Build history of the part. All positions in model axes, mm. A direction names the side the tool comes from. Give positions to 0.01 mm unless a question says otherwise; leave off trailing zeros. Order: outer loops, then holes, each group sorted by start corner. A loop starts at its lowest first (then second) coordinate and runs counter-clockwise, first axis right, second up. Notation, with made-up numbers: (20, 66) - (66, 66) arc R31 ccw to (66, 105) - close; hole circle Ø6 at (76.5, 54.25). An arc over 180 degrees is marked (long way). Use a Markdown table: item, result.
Autodesk Inventor part; units mm, degrees
ref_plane "Work Plane1" through (-19.467767, 1.0375, -4.375) normal (0, 0, -1) x (0, 1, 0)
ref_plane "YZ Plane" through (0, 0, 0) normal (1, 0, 0) x (0, 1, 0)
ref_plane "XZ Plane" through (0, 0, 0) normal (0, 1, 0) x (-1, 0, 0)
sketch "Sketch1" plane through (0, 0, 0) normal (0, 0, 1) x (1, 0, 0)
  circle A0 centre (1.767767, 26.667767) radius 7
  circle A1 centre (1.767767, 26.667767) radius 6.965
  circle A2 centre (1.767767, 26.667767) radius 6.09
  point P0 (0, 0)
  dimension "d0" = 0.035
  dimension "d2" = 0.875
ref_plane "Work Plane1" through (-19.467767, 1.0375, -4.375) normal (0, 0, -1) x (0, 1, 0)
sketch "Sketch1 outline for Extrusion1" plane through (0, 0, 0) normal (0, 0, 1) x (1, 0, 0)
  circle A0 centre (1.767767, 26.667767) radius 6.965
  circle A1 centre (1.767767, 26.667767) radius 6.09
extrude "Extrusion1" add sketch "Sketch1 outline for Extrusion1" along normal blind 1.25 from surface at -4.375
sketch "Sketch2" plane through (1.767767, 26.667767, -4.375) normal (0, 0, -1) x (-1, 0, 0)
  circle A0 centre (0, 0) radius 6.965
  circle A1 centre (0, 0) radius 6.09
  circle A2 centre (0, 0) radius 7.09
  circle A3 centre (0, 0) radius 9.09
  point P0 (1.767767, -26.667767)
  dimension "d5" = 0.125
  dimension "d6" = 2
extrude "Extrusion2" add sketch "Sketch2" along normal blind 1.25 contours A0 | A2 | A3
properties part number "Half Inch Lense Holder Cover (V5)"
1) Slice it at B-B (x = -2.5). Write the cut outline in (y, z) (3 decimals).
Computed:
| item | result |
|---|---|
| outline | (18.642, -5.625) - (22.323, -5.625) - (22.323, -3.125) - (21.163, -3.125) - (21.163, -4.375) - (18.642, -4.375) - close; (31.012, -5.625) - (34.694, -5.625) - (34.694, -4.375) - (32.172, -4.375) - (32.172, -3.125) - (31.012, -3.125) - close |
2) Tool access for faces 1 (the flat face through (6, 22, -3.125)), 2 (the flat face through (-3, 21, -4.375)): list every direction of +Z, -Z, +X, -X, +Y, -Y with a clear straight run to the whole face (end or side of a thin tool).
Computed:
| item | result |
|---|---|
| face 1 | +Z, +X, -X, +Y, -Y |
| face 2 | +Z |
3) Slice it at C-C (x = 8.25). Write the cut outline in (y, z) (3 decimals).
Computed:
| item | result |
|---|---|
| outline | (20.295, -5.625) - (33.04, -5.625) - (33.04, -4.375) - (29.216, -4.375) - (29.216, -3.125) - (24.12, -3.125) - (24.12, -4.375) - (20.295, -4.375) - close |
4) Wall check: line 1 (X direction, y = 26.5, z = -3.75); line 2 (Z direction, x = 8, y = 32) (3 decimals); line 3 (Y direction, x = 5.5, z = -5.15). Give the ranges that are in metal, low to high. Write a range as from..to.
Computed:
| item | result |
|---|---|
| line 1 | x = -5.2..-4.32, 7.86..8.73 |
| line 2 | z = -5.625..-4.375 |
| line 3 | y = 18.38..21.86, 31.48..34.96 |
5) Pin check, flat tips, straight feed: P1, Ø1, axis at x = 9, z = -5, coming from the +Y side; P2, Ø9.5, axis at x = 1.77, y = 26.67, coming from the +Z side; P3, Ø10, axis at x = 7, y = 33, coming from the +Z side (3 decimals); P4, Ø1, axis at y = 23, z = -5, coming from the +X side. Stop position of each tip, or through.
Computed:
| item | result |
|---|---|
| P1 | stops at y = 32.78 |
| P2 | passes through |
| P3 | stops at z = -3.125 |
| P4 | stops at x = 10.29 |
6) Slice it at A-A (y = 24.25). Write the cut outline in (x, z) (3 decimals), and give its area (3 significant figures).
Computed:
| item | result |
|---|---|
| outline | (-6.995, -5.625) - (-3.822, -5.625) - (-3.822, -3.125) - (-4.764, -3.125) - (-4.764, -4.375) - (-6.995, -4.375) - close; (7.357, -5.625) - (10.53, -5.625) - (10.53, -4.375) - (8.3, -4.375) - (8.3, -3.125) - (7.357, -3.125) - close |
| area | 10.3 mm² |
7) Slice it at D-D (z = -5.4). Write the cut outline in (x, y).
Computed:
| item | result |
|---|---|
| outline | circle Ø18.18 at (1.77, 26.67); hole circle Ø12.18 at (1.77, 26.67) |
